Design review of the part built by this model. Coordinates are the model's own, in mm. Give positions to 0.01 mm unless a question says otherwise; leave off trailing zeros. Loops run counter-clockwise (first coordinate to the right, second up) from the corner with the lowest first, then second, coordinate; pieces in that order, holes last. Notation, with made-up numbers: (19.25, 11.5) -> (27.25, 11.5) arc R31 cw to (27.25, 45.5) -> close; hole circle Ø9 at (-6.5, -5.75). An arc over 180 degrees is marked (long way). Use a Markdown table: item, result. Add a question column.
1. Add section C-C (y = -5). State the section outline as (x, z) points, and give its area (3 significant figures).
2. Add section A-A (x = 47). State the section outline as (y, z) points.
3. Add section D-D (x = 107.2). State the section outline as (y, z) points.
4. Add section B-B (z = 8.8). State the section outline as (x, y) points, and give its area (3 significant figures).
5. To check wall thickness, follow line 1 (X direction, y = -69.6, z = 8.8); line 2 (Y direction, x = 65, z = 2.3); line 3 (Z direction, x = 74, y = -15.5). State the ranges of each line that lie inside material, in increasing order.
6. For pin 1 Ø6 at (y, z) = (-18, 9) entering from +X; pin 2 Ø1.2 at (y, z) = (-71, 4) entering from -X; pin 3 Ø1.2 at (x, z) = (60, 2) entering from -Y; pin 4 Ø4 at (x, z) = (107, 11) entering from +Y, all flat-tipped, find the tip position at first contact; note any pin that passes through.
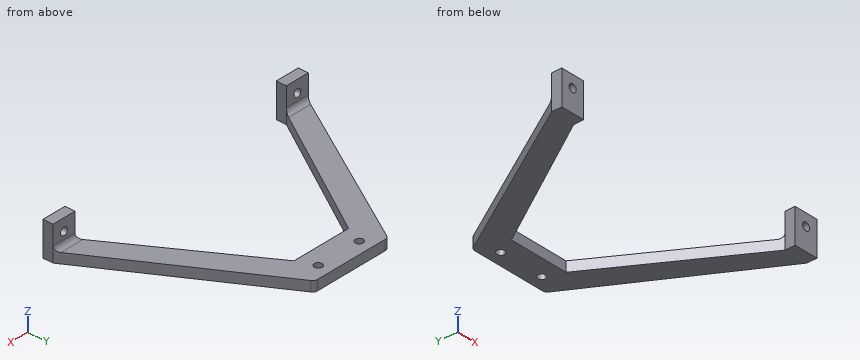
```python
from build123d import *

# Parameters (mm, degrees)
SKETCH1_W           = 112
SKETCH1_H           = 72
BOSS_EXTRUDE1_DEPTH = 4
SKETCH2_W           = 9.6
SKETCH2_H           = 4
BOSS_EXTRUDE2_DEPTH = 9.6
SKETCH3_R           = 1.55
CUT_EXTRUDE1_DEPTH  = 9.6
SKETCH4_R           = 1.55
CUT_EXTRUDE2_DEPTH  = 9.6
CUT_EXTRUDE4_DEPTH  = 9.6
CUT_EXTRUDE5_DEPTH  = 9.6
CUT_EXTRUDE6_DEPTH  = 10
FILLET1_R           = 2
FILLET2_R           = 2


with BuildPart() as part:
    # Sketch1 → Boss-Extrude1 (new body)
    with BuildSketch(Plane.XY):
        with Locations((56, -36)):
            Rectangle(SKETCH1_W, SKETCH1_H)
    extrude(amount=BOSS_EXTRUDE1_DEPTH)

    # Sketch2 → Boss-Extrude2 (add)
    with BuildSketch(Plane.XY.offset(4)):
        with Locations((4.8, -70)):
            Rectangle(SKETCH2_W, SKETCH2_H)
        with Locations((107.2, -70)):
            Rectangle(SKETCH2_W, SKETCH2_H)
        with Locations((56, -70)):
            Rectangle(SKETCH2_W, SKETCH2_H)
    extrude(amount=BOSS_EXTRUDE2_DEPTH)

    # Sketch3 → Cut-Extrude1 (cut)
    with BuildSketch(Plane(origin=(0, -68, 0), x_dir=(1, 0, 0), z_dir=(0, 1, 0))):
        with Locations(Location((4.8, -8.8, 0), (0, 0, 270))):
            Circle(SKETCH3_R)
        with Locations(Location((56, -8.8, 0), (0, 0, 270))):
            Circle(SKETCH3_R)
        with Locations(Location((107.2, -8.8, 0), (0, 0, 270))):
            Circle(SKETCH3_R)
    extrude(amount=-CUT_EXTRUDE1_DEPTH, mode=Mode.SUBTRACT)

    # Sketch4 → Cut-Extrude2 (cut)
    with BuildSketch(Plane.XY.offset(4)):
        with Locations((47, -5)):
            Circle(SKETCH4_R)
        with Locations((65, -5)):
            Circle(SKETCH4_R)
        with Locations((56, -14)):
            Circle(SKETCH4_R)
    extrude(amount=-CUT_EXTRUDE2_DEPTH, mode=Mode.SUBTRACT)

    # Sketch5 → Cut-Extrude4 (cut)
    with BuildSketch(Plane.XY.offset(4)):
        Polygon((0, -68), (0, 0), (40, 0), align=None)
        Polygon((72, 0), (112, -68), (112, 0), align=None)
    extrude(amount=-CUT_EXTRUDE4_DEPTH, mode=Mode.SUBTRACT)

    # Sketch6 → Cut-Extrude5 (cut)
    with BuildSketch(Plane.XY.offset(4)):
        Polygon((9.6, -68), (44, -12), (51.2, -68), (51.2, -72), (9.6, -72), align=None)
        Polygon((102.4, -72), (102.4, -68), (68, -12), (60.8, -68), (60.8, -72), align=None)
    extrude(amount=-CUT_EXTRUDE5_DEPTH, mode=Mode.SUBTRACT)

    # Sketch7 → Cut-Extrude6 (cut)
    with BuildSketch(Plane.XY.offset(4)):
        Polygon((44, -12), (68, -12), (68, -81.921915354), (38.62828306, -80.469678764), align=None)
    extrude(amount=-CUT_EXTRUDE6_DEPTH, mode=Mode.SUBTRACT)


with BuildPart() as body_2:
    # of the pieces the cut leaves, the one that is kept (cut_extrude6_keep)
    add(part.part.solids().sort_by_distance((40, 0, 0))[0])

    # Fillet1
    fillet1_edges = [body_2.edges().sort_by_distance(p)[0] for p in [
        (4.8, -68, 4),
        (107.2, -68, 4),
    ]]
    fillet(fillet1_edges, radius=FILLET1_R)

    # Fillet2
    fillet2_edges = [body_2.edges().sort_by_distance(p)[0] for p in [
        (40, 0, 2),
        (72, 0, 2),
    ]]
    fillet(fillet2_edges, radius=FILLET2_R)


solid = body_2.part
```
Taken from the geometry:
| question | item | result |
|---|---|---|
| 1 | outline | (37.06, 0) -> (45.45, 0) -> (45.45, 4) -> (37.06, 4) -> close; (48.55, 0) -> (63.45, 0) -> (63.45, 4) -> (48.55, 4) -> close; (66.55, 0) -> (74.94, 0) -> (74.94, 4) -> (66.55, 4) -> close |
| 1 | area | 127 mm^2 |
| 2 | outline | (-12, 0) -> (-6.55, 0) -> (-6.55, 4) -> (-12, 4) -> close; (-3.45, 0) -> (0, 0) -> (0, 4) -> (-3.45, 4) -> close |
| 3 | outline | (-72, 0) -> (-59.84, 0) -> (-59.84, 4) -> (-66, 4) arc R2 cw to (-68, 6) -> (-68, 7.25) -> (-72, 7.25) -> close; (-72, 10.35) -> (-68, 10.35) -> (-68, 13.6) -> (-72, 13.6) -> close |
| 4 | outline | (0, -72) -> (3.25, -72) -> (3.25, -68) -> (0, -68) -> close; (6.35, -72) -> (9.6, -72) -> (9.6, -68) -> (6.35, -68) -> close; (102.4, -72) -> (105.65, -72) -> (105.65, -68) -> (102.4, -68) -> close; (108.75, -72) -> (112, -72) -> (112, -68) -> (108.75, -68) -> close |
| 4 | area | 52.0 mm^2 |
| 5 | line 1 | x = 0 to 3.25, 6.35 to 9.6, 102.4 to 105.65, 108.75 to 112 |
| 5 | line 2 | y = -12 to -6.55, -3.45 to 0 |
| 5 | line 3 | z = 0 to 4 |
| 6 | pin 1 | passes through |
| 6 | pin 2 | stops at x = 0 |
| 6 | pin 3 | stops at y = -12 |
| 6 | pin 4 | stops at y = -68 |
